CAD build for the part. Positions are in the model's coordinates, mm. Coordinates: 2 decimals unless noted, no trailing zeros. Write each loop counter-clockwise with the first axis right and the second up, starting at its lowest first coordinate (ties: lowest second). Pieces come first, ordered by that corner, then holes. Notation, with made-up numbers: (11, 43.5) -> (24, 43.5) arc R25 cw to (24, 66.5) -> close; hole circle Ø7 at (76.5, 72.5). An arc over 180 degrees is marked (long way). Answer as CSV lines item,"result".
```python
from build123d import *

# Parameters (mm, degrees)
BOSS_EXTRUDE1_DEPTH = 238
SKETCH3_W           = 15
SKETCH3_H           = 15
CUT_EXTRUDE1_DEPTH  = 54
FILLET1_R           = 0.5


with BuildPart() as part:
    # Sketch2 → Boss-Extrude1 (new body)
    with BuildSketch(Plane.XY.offset(-3)):
        with BuildLine():
            Line((446.391965645, 20.11245238), (474.43313548, 20.11245238))
            Line((474.43313548, 20.11245238), (447.390900992, 27.530319971))
            ThreePointArc((447.390900992, 27.530319971), (442.649552271, 24.39262378), (446.391965645, 20.11245238))
        make_face()
    extrude(amount=BOSS_EXTRUDE1_DEPTH)

    # Sketch3 → Cut-Extrude1 (cut)
    with BuildSketch(Plane.XZ.offset(30.589717262)):
        with Locations((450.115770482, 182.5)):
            Rectangle(SKETCH3_W, SKETCH3_H)
        with Locations((450.115770482, 49.5)):
            Rectangle(SKETCH3_W, SKETCH3_H)
    extrude(amount=-CUT_EXTRUDE1_DEPTH, mode=Mode.SUBTRACT)

    # Fillet1
    fillet1_edges = [part.edges().sort_by_distance(p)[0] for p in [
        (474.43313548, 20.11245238, 116),
    ]]
    fillet(fillet1_edges, radius=FILLET1_R)


solid = part.part
```
Item 1: Wall check: line 1 (Z direction, x = 446, y = 22); line 2 (Y direction, x = 461.5, z = 120); line 3 (Y direction, x = 469, z = 124). Give the ranges that are in metal, low to high. Write a range as from..to.
Answer below:
line 1,"z = -3..42, 57..175, 190..235"
line 2,"y = 20.11..23.66"
line 3,"y = 20.11..21.6"
Item 2: Saw through at A-A on z = 113. Give the cut face in (x, y).
Answer below:
outline,"(446.39, 20.11) -> (470.72, 20.11) arc R0.5 ccw to (470.85, 21.09) -> (447.39, 27.53) arc R3.78 ccw (long way) to start"
Item 3: Saw through at B-B on y = 24.75. Give the cut face in (x, z), and give its area (3 significant figures).
Answer below:
outline,"(442.72, -3) -> (457.53, -3) -> (457.53, 235) -> (442.72, 235) -> close"
area,"3,530 mm2"
Item 4: Two-plate mould, pull along Z, no slides. Class faces 1 (the flat face through (450, 23.41, 183)), 2 (the flat face through (450, 23.41, 50)), 3 (the flat face through (454, 23, 235)), 4 (the flat face through (454, 23, -3)): pulls with the +Z half, pulls with the -Z half, needs draft (parallel to the pull), parting line crosses it, or undercut.
Answer below:
face 1,"undercut"
face 2,"undercut"
face 3,"pulls with the +Z half"
face 4,"pulls with the -Z half"
Item 5: Flat gauge pins, fed straight in: pin 1 (2 mm diameter, centred on x = 467, z = 150.5, fed in from +Y); pin 2 (4.5 mm diameter, centred on x = 449.5, z = 50.5, fed in from -Y); pin 3 (1.6 mm diameter, centred on y = 21.5, z = 183, fed in from -X). Where does each tip first touch, or does it go through?
Answer below:
pin 1,"stops at y = 22.43"
pin 2,"stops at y = 23.41"
pin 3,"stops at x = 457.62"
